from build123d import *

# Parameters (mm, degrees)
BOSS_EXTRU_2_DEPTH       = 10
ENL_V_MAT_EXTRU_25_DEPTH = 7
ESQUISSE5_W              = 37.59862274
ESQUISSE5_H              = 68.527189437
ENL_V_MAT_EXTRU_26_DEPTH = 6


with BuildPart() as part:
    # Esquisse2 → Boss.-Extru.2 (new body)
    with BuildSketch(Plane.XY):
        Polygon((0, 64.5), (0, -68.5), (11, -58), (11, 75), align=None)
    extrude(amount=BOSS_EXTRU_2_DEPTH)

    # Esquisse4 → Enlèv. mat.-Extru.25 (cut)
    with BuildSketch(Plane.XY.offset(10)):
        Polygon((2.407262121, 3.056563683), (2.407262121, 9.256563683), (8.6, 8.956567739), (8.6, 2.756567739), align=None)
    extrude(amount=-ENL_V_MAT_EXTRU_25_DEPTH, mode=Mode.SUBTRACT)

    # Esquisse5 → Enlèv. mat.-Extru.26 (cut)
    with BuildSketch(Plane.XY.offset(10)):
        with Locations((3.383685942, 50.502193636)):
            Rectangle(ESQUISSE5_W, ESQUISSE5_H)
        with Locations((3.383685942, -38.789058157)):
            Rectangle(ESQUISSE5_W, ESQUISSE5_H)
    extrude(amount=-ENL_V_MAT_EXTRU_26_DEPTH, mode=Mode.SUBTRACT)


solid = part.part
Part model, mm, in its own coordinate system. A direction names the side the tool comes from. Give positions to 0.01 mm unless a question says otherwise; leave off trailing zeros. Order: outer loops, then holes, each group sorted by start corner. A loop starts at its lowest first (then second) coordinate and runs counter-clockwise, first axis right, second up. Notation, with made-up numbers: (11.25, -26) - (47.25, -26) arc R33 cw to (47.25, 6) - close; hole circle Ø8 at (85.25, 45). An arc over 180 degrees is marked (long way). Use a Markdown table: item, result.
1) Saw through at C-C on y = -41. List the corners of the cut face in (x, z), plus the area to 3 significant figures.
Checked values:
| item | result |
|---|---|
| outline | (0, 0) - (11, 0) - (11, 4) - (0, 4) - close |
| area | 44.0 mm² |
2) Saw through at B-B on x = 1.25. List the corners of the cut face in (y, z), plus the area to 3 significant figures.
Checked values:
| item | result |
|---|---|
| outline | (-67.31, 0) - (65.69, 0) - (65.69, 4) - (16.24, 4) - (16.24, 10) - (-4.53, 10) - (-4.53, 4) - (-67.31, 4) - close |
| area | 657 mm² |
3) Flat gauge pins, fed straight in: P1, Ø3.5, axis at x = 4.5, y = 35, coming from the +Z side; P2, Ø5, axis at x = 8, z = 5.5, coming from the -Y side; P3, Ø1.5, axis at x = 9.5, z = 3.5, coming from the -Y side. Where does each tip first touch, or does it go through?
Checked values:
| item | result |
|---|---|
| P1 | z = 4 |
| P2 | y = -62.77 |
| P3 | y = -60.15 |
4) Saw through at A-A on z = 8.25. List the corners of the cut face in (x, y).
Checked values:
| item | result |
|---|---|
| outline | (0, -4.53) - (11, -4.53) - (11, 16.24) - (0, 16.24) - close; hole (2.41, 3.06) - (8.6, 2.76) - (8.6, 8.96) - (2.41, 9.26) - close |
5) 3-axis set-ups, long thin cutter, end or side, ignore diameter. For faces 1 (the flat face through (5, 46, 4)), 2 (the flat face through (5.547, 2.904, 6.549)), 3 (the flat face through (5, -4.525, 7)): which of +Z, -Z, +X, -X, +Y, -Y reach the whole face in a straight line?
Checked values:
| item | result |
|---|---|
| face 1 | +Z, +X, -X, +Y |
| face 2 | +Z |
| face 3 | +Z, +X, -X, -Y |
6) Two-plate mould, pull along X, no slides. Class faces 4 (the flat face through (5.46, 9.11, 6.55)), 5 (the flat face through (0, -1, 3)), 6 (the flat face through (5, 16.239, 7)), 7 (the flat face through (2.407, 6, 7)): +X half, -X half, draft (parallel to the pull), parting line (faces both ways), or undercut.
Checked values:
| item | result |
|---|---|
| face 4 | undercut |
| face 5 | -X half |
| face 6 | draft |
| face 7 | undercut |
7) Probe L1, parallel to Y at x = 9, z = 4.75; L2, parallel to Z at x = 4.25, y = -12.5; L3, parallel to Y at x = 4.75, z = 4.25. List the from-to ranges inside material, lowest first. Write a range as from..to.
Checked values:
| item | result |
|---|---|
| L1 | -4.53..16.24 |
| L2 | 0..4 |
| L3 | -4.53..2.94, 9.14..16.24 |
